For this review, take the finished solid that the model builds, in its own axes (mm). Face numbers are marked on the shaded views. A direction names the side the tool comes from. Give positions to 0.01 mm unless a question says otherwise; leave off trailing zeros. Write each loop counter-clockwise with the first axis right and the second up, starting at its lowest first coordinate (ties: lowest second). Pieces come first, ordered by that corner, then holes.
Q1. Machinability: for the marked faces 1 and 2, which of the approach directions +Z, -Z, +X, -X, +Y, -Y give a long, thin tool a straight path to every point of the face, cutting with its end or side? Answer none if there is none.
Q2. Insertion check: P1, Ø1.5, axis at y = 11.5, z = -6, coming from the -X side; P2, Ø1, axis at x = -15, z = -3, coming from the +Y side; P3, Ø12, axis at y = -4, z = -55, coming from the -X side. Each pin has a flat end and moves straight along its axis. Give the tip position at first contact, or say it passes through.
Q3. For line 1 (X direction, y = 0, z = -40); line 2 (Y direction, x = 0, z = 14), list the stretches that pass through material, from the lowest coordinate up.
Q4. We need section A-A (z = -37). Write out the cut boundary in (x, y), then the cut area to 3 significant figures.
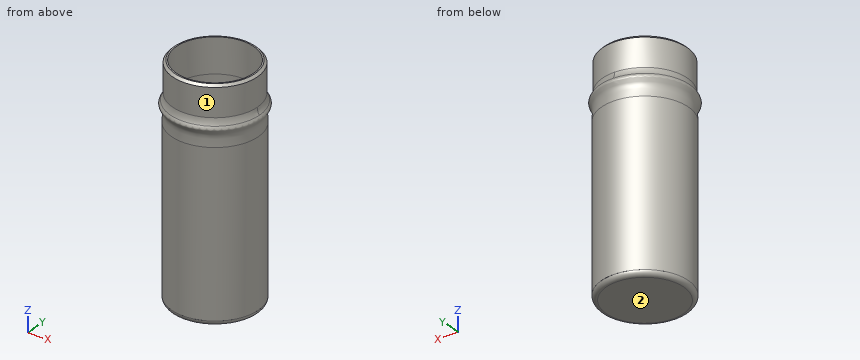
Autodesk Inventor part; units mm, degrees
ref_plane "YZ Plane" through (0, 0, 0) normal (1, 0, 0) x (0, 1, 0)
ref_plane "XZ Plane" through (0, 0, 0) normal (0, 1, 0) x (-1, 0, 0)
ref_plane "XY Plane" through (0, 0, 0) normal (0, 0, 1) x (1, 0, 0)
sketch "Skizze1" plane through (0, 0, 0) normal (0, 0, 1) x (1, 0, 0)
  circle A0 centre (0, 0) radius 18.75
  circle A1 centre (0, 0) radius 16.75
  dimension "d0" = 37.5
  dimension "d1" = 2
extrude "Extrusion1" add sketch "Skizze1" against normal blind 70
sketch "Skizze2" plane through (0, 0, -70) normal (0, 0, -1) x (-1, 0, 0)
  circle A0 centre (0, 0) radius 18.75
extrude "Extrusion2" add sketch "Skizze2" along normal blind 2
fillet "Rundung1" radius 2 2 edges at (-16.75, 0, -70) (18.75, 0, -72)
sketch "Skizze3" plane through (0, 0, 0) normal (1, 0, 0) x (0, 1, 0)
  line L0 (18.75, 0) -> (18.75, -70)
  line L1 (-18.75, 0) -> (18.75, 0)
  line L2 (-16.75, 0) -> (16.75, 0)
  line L3 (18.75, 0) -> (16.75, 0)
  line L4 (16.75, 0) -> (16.75, 10)
  line L5 (16.75, 10) -> (18.35, 10)
  spline S0 degree 4 poles (18.35, 10) (22.5236, 5.438) (17.0645, 8.0767) (18.75, 3.082) (18.75, 0) knots 0 0 0 0 0 1 1 1 1 1
  line L6 (0, -86.0201) -> (0, 26.1206)
  point P0 (0, 0)
  point P1 (19.65, 6.8)
  point P2 (18.75, 5)
  dimension "d7" = 10
  dimension "d8" = 1.6
  dimension "d9" = 2
  dimension "d10" = 2.9
  dimension "d11" = 3.2
  dimension "d12" = 5
revolve "Umdrehung1" add sketch "Skizze3" angle 360 about axis through (0, 0, -10) along (0, 0, 1)
sketch "Skizze4" plane through (0, 0, 10) normal (0, 0, 1) x (1, 0, 0)
  circle A0 centre (0, 0) radius 18.35
  circle A1 centre (0, 0) radius 16.75
  point P0 (0, 18.35)
extrude "Extrusion3" add sketch "Skizze4" along normal blind 15
fillet "Rundung2" radius 5 2 edges at (12.9754, 12.9754, 10) (-12.9754, -12.9754, 10)
chamfer "Fase1" distance 1 angle 45 1 edges at (-18.35, 0, 25)
equation "\"G_L\" = 0"
equation "\"G_H\" = 0"
equation "\"G_B\" = 0"
properties part number "Löffelbox_unten" material "GEDA Stahl"
Computed:
1. face 1: +Z
1. face 2: -Z, +X, -X, +Y, -Y
2. P1: stops at x = -15.36
2. P2: stops at y = 11.89
2. P3: stops at x = -18.75
3. line 1: x = -18.75 to -16.75, 16.75 to 18.75
3. line 2: y = -18.35 to -16.75, 16.75 to 18.35
4. outline: circle Ø37.5 at (0, 0); hole circle Ø33.5 at (0, 0)
4. area: 223 mm2
